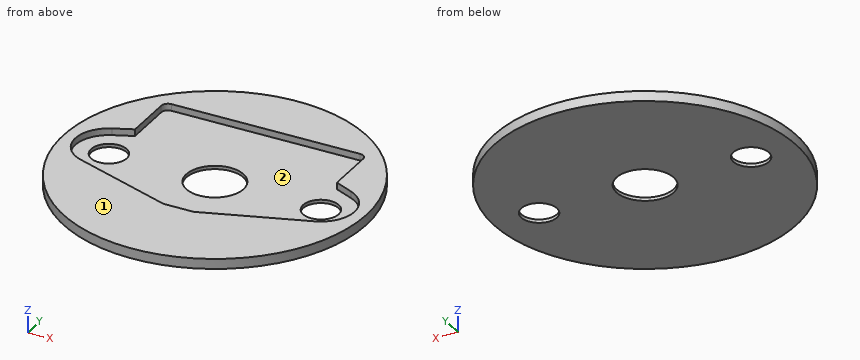
```python
from build123d import *

# Parameters (mm, degrees)
SKETCH_R      = 22.5
PAD_DEPTH     = 1
SKETCH001_R   = 22.5
PAD001_DEPTH  = 0.5
SKETCH002_R   = 4.25
SKETCH002_R_2 = 2.65
POCKET_DEPTH  = 1.501
FILLET_R      = 1
FILLET001_R   = 1


with BuildPart() as part:
    # Sketch → Pad (new body)
    with BuildSketch(Plane.XY):
        Circle(SKETCH_R)
        with BuildLine():
            ThreePointArc((17.39553, -4.721465), (20.746006, -0.199818), (17.767345, 4.574967))
            Line((15, 5.795235), (17.767345, 4.574967))
            Line((15, 14), (15, 5.795235))
            Line((-15, 14), (15, 14))
            Line((-15, 14), (-15, 5.795235))
            Line((-17.767345, 4.574967), (-15, 5.795235))
            ThreePointArc((-17.767345, 4.574967), (-20.746006, -0.199818), (-17.39553, -4.721465))
            Line((-17.39553, -4.721465), (-2.25, -10))
            Line((-2.25, -10), (2.25, -10))
            Line((17.39553, -4.721465), (2.25, -10))
        make_face(mode=Mode.SUBTRACT)
    extrude(amount=PAD_DEPTH)

    # Sketch001 (on Face12 of Pad) → Pad001 (join)
    with BuildSketch(Plane(origin=(0, 0, 0), x_dir=(1, 0, 0), z_dir=(0, 0, -1))):
        Circle(SKETCH001_R)
    extrude(amount=PAD001_DEPTH)

    # Sketch002 (on Face4 of Pad001) → Pocket (cut, through all)
    with BuildSketch(Plane(origin=(0, 0, -0.5), x_dir=(1, 0, 0), z_dir=(0, 0, -1))):
        Circle(SKETCH002_R)
        with Locations((-15.75, 0)):
            Circle(SKETCH002_R_2)
        with Locations((15.75, 0)):
            Circle(SKETCH002_R_2)
    extrude(amount=-POCKET_DEPTH, mode=Mode.SUBTRACT)

    # Fillet
    fillet_edges = [part.edges().sort_by_distance(p)[0] for p in [
        (15, 14, 0.5),
        (-15, 14, 0.5),
    ]]
    fillet(fillet_edges, radius=FILLET_R)

    # Fillet001
    fillet001_edges = [part.edges().sort_by_distance(p)[0] for p in [
        (-2.25, -10, 0.5),
        (2.25, -10, 0.5),
    ]]
    fillet(fillet001_edges, radius=FILLET001_R)


solid = part.part
```
The listing builds one solid part. Answer for the finished solid, in the listing's coordinates (mm). Face numbers are marked on the shaded views. Give positions to 0.01 mm unless a question says otherwise; leave off trailing zeros. Order: outer loops, then holes, each group sorted by start corner. A loop starts at its lowest first (then second) coordinate and runs counter-clockwise, first axis right, second up. Notation, with made-up numbers: (88, 75.25) - (93, 75.25) arc R10 cw to (93, 84.25) - close; hole circle Ø11 at (38.5, 57). An arc over 180 degrees is marked (long way). Use one line per item in the form item = value. Start each with the question number.
(1) A cutting plane is placed at C-C, the plane z = 0.6. Write down the section's boundary in (x, y).
(2) Consider line 1 (X direction, y = 0, z = -0.15); line 2 (Y direction, x = 0, z = -0.2); line 3 (Y direction, x = 15.75, z = -0.3). Determine where each line is inside the solid, lowest interval first. Write a range as from..to.
(3) The mould has two halves that part along X. Classify the marked faces 1 and 2: released by +X, released by -X, zero draft, split by the parting line, or undercut.
(4) A cutting plane is placed at A-A, the plane x = 0. Write down the section's boundary in (y, z).
(5) A cutting plane is placed at D-D, the plane x = 11. Write down the section's boundary in (y, z).
(6) Flat-ended cylindrical pins translate along their axes: pin 1 Ø7 at (x, y) = (6, 3) entering from +Z; pin 2 Ø8 at (x, y) = (17.5, 2.5) entering from +Z; pin 3 Ø0.8 at (y, z) = (10, 0.5) entering from +X. Find the tip coordinate at first contact, or state that the pin passes through.
(7) A cutting plane is placed at B-B, the plane y = 0. Write down the section's boundary in (x, z), then the cut area to 4 significant figures.
Ans:
q1.outline = circle Ø45 at (0, 0); hole (-17.77, 4.57) arc R5 ccw to (-17.4, -4.72) - (-2.41, -9.94) arc R1 ccw to (-2.08, -10) - (2.08, -10) arc R1 ccw to (2.41, -9.94) - (17.4, -4.72) arc R5 ccw to (17.77, 4.57) - (15, 5.8) - (15, 13) arc R1 ccw to (14, 14) - (-14, 14) arc R1 ccw to (-15, 13) - (-15, 5.8) - close
q2.line_1 = -22.5..-18.4, -13.1..-4.25, 4.25..13.1, 18.4..22.5
q2.line_2 = -22.5..-4.25, 4.25..22.5
q2.line_3 = -16.07..-2.65, 2.65..16.07
q3.face_1 = zero draft
q3.face_2 = undercut
q4.outline = (-22.5, -0.5) - (-4.25, -0.5) - (-4.25, 0) - (-10, 0) - (-10, 1) - (-22.5, 1) - close; (4.25, -0.5) - (22.5, -0.5) - (22.5, 1) - (14, 1) - (14, 0) - (4.25, 0) - close
q5.outline = (-19.63, -0.5) - (19.63, -0.5) - (19.63, 1) - (14, 1) - (14, 0) - (-6.95, 0) - (-6.95, 1) - (-19.63, 1) - close
q6.pin_1 = 0
q6.pin_2 = 1
q6.pin_3 = 20.35
q7.outline = (-22.5, -0.5) - (-18.4, -0.5) - (-18.4, 0) - (-20.75, 0) - (-20.75, 1) - (-22.5, 1) - close; (-13.1, -0.5) - (-4.25, -0.5) - (-4.25, 0) - (-13.1, 0) - close; (4.25, -0.5) - (13.1, -0.5) - (13.1, 0) - (4.25, 0) - close; (18.4, -0.5) - (22.5, -0.5) - (22.5, 1) - (20.75, 1) - (20.75, 0) - (18.4, 0) - close
q7.area = 16.45 mm^2
